Here's the drawing with two shaded views (mm, measured from the low corner). I have some questions. A direction names the side the tool comes from. Give positions to 0.01 mm unless a question says otherwise; leave off trailing zeros. Loops run counter-clockwise (first coordinate to the right, second up) from the corner with the lowest first, then second, coordinate; pieces in that order, holes last.
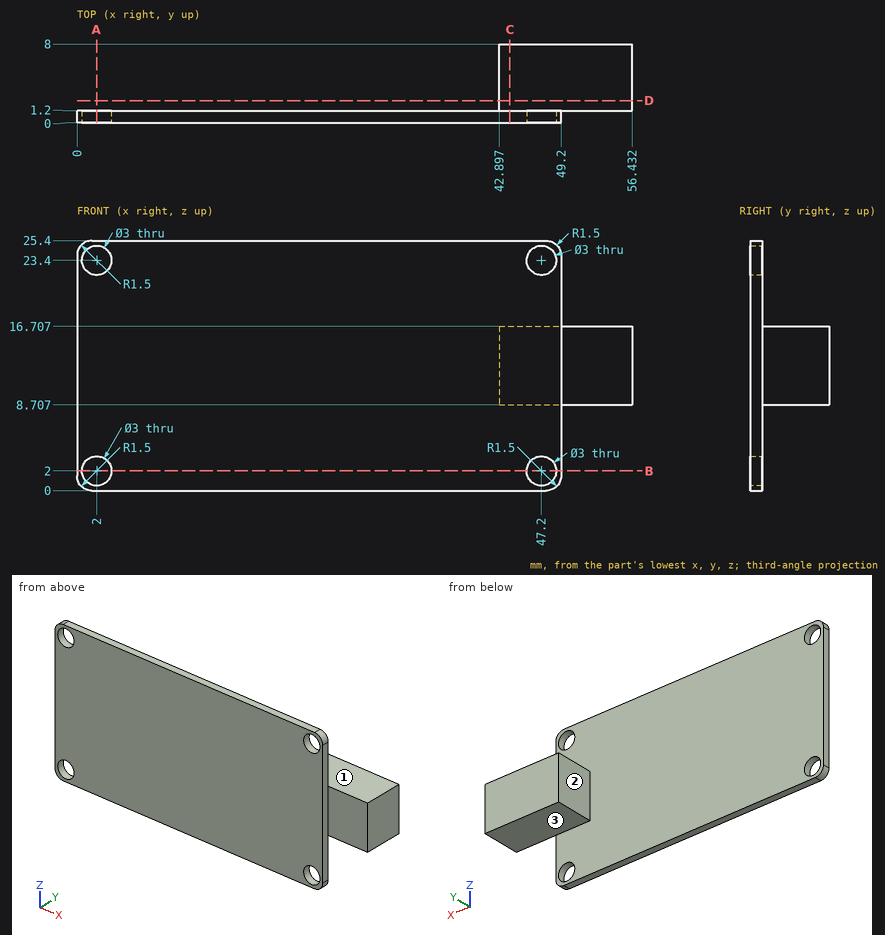
(1) Please list where these lines run through material, in increasing order: probe 1 along X at (y, z) = (0.45, 23.4); probe 2 along Y at (x, z) = (16, 10.5); probe 3 along X at (y, z) = (1.5, 11).
Returned:
probe 1: x = 0 to 0.5, 3.5 to 45.7, 48.7 to 49.2
probe 2: y = 0 to 1.2
probe 3: x = 42.9 to 56.43
(2) Suppose I cut it at D-D on y = 2.25. List the corners of the cut face in (x, z) for me.
Returned:
outline: (42.9, 8.71) - (56.43, 8.71) - (56.43, 16.71) - (42.9, 16.71) - close
(3) Which directions (+Z, -Z, +X, -X, +Y, -Y) give clear straight access to the entire face, cutting with the end or side of a thin tool? Please do the marked faces 1, 2 and 3.
Returned:
face 1: +Z, +X, -X, +Y
face 2: +Z, -Z, -X, +Y
face 3: -Z, +X, -X, +Y
(4) Suppose I cut it at A-A on x = 2. List the corners of the cut face in (y, z) for me.
Returned:
outline: (0, 0) - (1.2, 0) - (1.2, 0.5) - (0, 0.5) - close; (0, 3.5) - (1.2, 3.5) - (1.2, 21.9) - (0, 21.9) - close; (0, 24.9) - (1.2, 24.9) - (1.2, 25.4) - (0, 25.4) - close
(5) Suppose I cut it at B-B on z = 2. List the corners of the cut face in (x, y) for me.
Returned:
outline: (0, 0) - (0.5, 0) - (0.5, 1.2) - (0, 1.2) - close; (3.5, 0) - (45.7, 0) - (45.7, 1.2) - (3.5, 1.2) - close; (48.7, 0) - (49.2, 0) - (49.2, 1.2) - (48.7, 1.2) - close
(6) Will these pins go through, and if not, where does the flat tip stop? P1, Ø5, axis at x = 47.2, z = 23.4, coming from the +Y side; P2, Ø2, axis at x = 51, y = 3, coming from the -Z side; P3, Ø6, axis at x = 52.5, z = 13.5, coming from the -Y side.
Returned:
P1: stops at y = 1.2
P2: stops at z = 8.71
P3: stops at y = 1.2
(7) Suppose I cut it at C-C on x = 44. List the corners of the cut face in (y, z) for me.
Returned:
outline: (0, 0) - (1.2, 0) - (1.2, 8.71) - (8, 8.71) - (8, 16.71) - (1.2, 16.71) - (1.2, 25.4) - (0, 25.4) - close
